Here's how the part is built. I have some questions about the finished solid (model axes, mm). Round coordinates to 2 decimals unless told otherwise and drop trailing zeros. Loops run counter-clockwise (first coordinate to the right, second up) from the corner with the lowest first, then second, coordinate; pieces in that order, holes last. Notation, with made-up numbers: M -27.75,39 L -2.75,39 A8 ccw -2.75,50 Z; hole C 73,-10 d3. An arc over 180 degrees is marked long. One line per question, with ' | ' between items. Start each with the question number.
```python
from build123d import *

# Parameters (mm, degrees)
F1_DEPTH = 30
F2_R     = 1.65
F3_DEPTH = 5.6
F5_DEPTH = 0.8


with BuildPart() as f1:
    # F0 (on Right) → F1 (new body)
    with BuildSketch(Plane.YZ):
        Polygon((-20, 5.6), (-20, 0), (20, 0), (20, 1.6), (0, 1.6), (0, 4), (20, 4), (20, 5.6), align=None)
    extrude(amount=F1_DEPTH)

    # F2 (on face) → F3 (cut, through all)
    with BuildSketch(Plane.XY.offset(5.6)):
        with Locations((7.5, 10)):
            Circle(F2_R)
        with Locations((22.5, 10)):
            Circle(F2_R)
    extrude(amount=-F3_DEPTH, mode=Mode.SUBTRACT)

    # F4 (on face) → F5 (cut)
    with BuildSketch(Plane(origin=(0, 0, 0), x_dir=(1, 0, 0), z_dir=(0, 0, -1))):
        Polygon((25.733162, -10), (24.116581, -7.2), (20.883419, -7.2), (19.266838, -10), (20.883419, -12.8), (24.116581, -12.8), align=None)
        Polygon((10.733162, -10), (9.116581, -7.2), (5.883419, -7.2), (4.266838, -10), (5.883419, -12.8), (9.116581, -12.8), align=None)
    extrude(amount=-F5_DEPTH, mode=Mode.SUBTRACT)


solid = f1.part
```
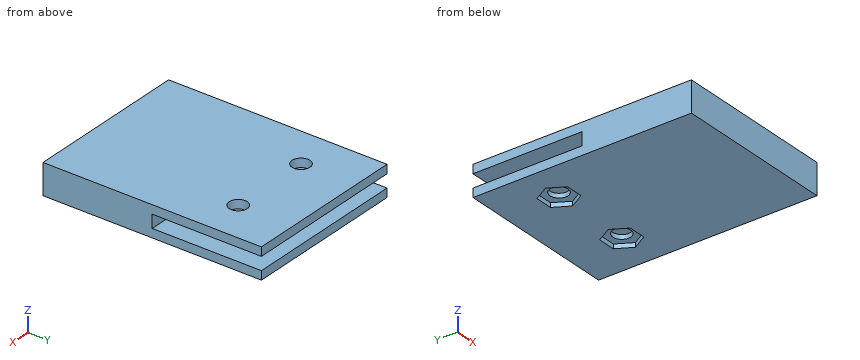
1) Please list where these lines run through material, in increasing order: L1, parallel to Z at x = 12.25, y = 16.5; L2, parallel to Y at x = 7.5, z = 4.35; L3, parallel to Z at x = 9.25, y = 11. Write a range as from..to.
2) Imagine slicing it at B-B (y = 16.5). Write out the boundary of the cut face in (x, z).
3) Imagine slicing it at A-A (x = 7.5). Write out the boundary of the cut face in (y, z), then the cut area to 3 significant figures.
4) Imagine slicing it at D-D (y = 9). State how many separate pieces and enclosed holes the cut face has, then the cut area to 3 significant figures.
5) I'm going to push a flat-ended pin straight in: pin 1 Ø3 at (x, y) = (6.5, 9.5) entering from -Z. Where does the tip first touch, or does it pass through?
6) Imagine slicing it at C-C (x = 13). Write out the boundary of the cut face in (y, z), then the cut area to 3 significant figures.
Results are:
1) L1: 0..1.6, 4..5.6 | L2: -20..8.35, 11.65..20 | L3: 0.8..1.6, 4..5.6
2) outline: M 0,0 L 30,0 L 30,1.6 L 0,1.6 Z; M 0,4 L 30,4 L 30,5.6 L 0,5.6 Z
3) outline: M -20,0 L 7.2,0 L 7.2,0.8 L 8.35,0.8 L 8.35,1.6 L 0,1.6 L 0,4 L 8.35,4 L 8.35,5.6 L -20,5.6 Z; M 11.65,0.8 L 12.8,0.8 L 12.8,0 L 20,0 L 20,1.6 L 11.65,1.6 Z; M 11.65,4 L 20,4 L 20,5.6 L 11.65,5.6 Z | area: 164 mm²
4) separate pieces: 6 | enclosed holes: 0 | area: 74.9 mm²
5) pin 1: z = 0.8
6) outline: M -20,0 L 20,0 L 20,1.6 L 0,1.6 L 0,4 L 20,4 L 20,5.6 L -20,5.6 Z | area: 176 mm²
